Model file for the job. Use its own axes, mm. Face numbers are marked on the shaded views. A direction names the side the tool comes from. Round coordinates to 2 decimals unless told otherwise and drop trailing zeros. Order: outer loops, then holes, each group sorted by start corner. A loop starts at its lowest first (then second) coordinate and runs counter-clockwise, first axis right, second up. Notation, with made-up numbers: M 21,24 L 27,24 A9 cw 27,37 Z; hole C 60.5,3 d7. An arc over 180 degrees is marked long. Return JSON: item names as keys, results as strings. Group by question number.
Item 1: Probe line 1 along Y through (x, z) = (-6, 0); line 2 along X through (y, z) = (44, 25.5); line 3 along Y through (x, z) = (-37, -0.5). List the from-to ranges inside material, lowest first.
Item 2: Slice it at D-D on z = 40. Write the cut outline in (x, y), then the cut area to 3 significant figures.
Item 3: Slice it at C-C on y = 37.5. Write the cut outline in (x, z).
Item 4: Slice it at B-B on x = 0. Write the cut outline in (y, z), then the cut area to 3 significant figures.
Item 5: Slice it at A-A on z = 0. Write the cut outline in (x, y).
Item 6: Pin check, flat tips, straight feed: pin 1 Ø3 at (y, z) = (77.5, -16.5) entering from -X; pin 2 Ø1.5 at (x, z) = (39.5, -0.5) entering from -Y; pin 3 Ø2 at (y, z) = (43, 40) entering from -X; pin 4 Ø12 at (x, y) = (-25, 19.5) entering from +Z. Stop position of each tip, or through.
Item 7: Which spindle directions (+Z, -Z, +X, -X, +Y, -Y) get a long thin tool onto all of the face, cutting with end or side? Do the marked faces 1, 2, 3, 4 and 5. Say none if no direction does.
from build123d import *

# Parameters (mm, degrees)
SKETCH1_R           = 50
BOSS_EXTRUDE1_DEPTH = 10
SKETCH2_W           = 50
SKETCH2_H           = 75
BOSS_EXTRUDE2_DEPTH = 80
SKETCH3_R           = 25
CUT_EXTRUDE4_DEPTH  = 76
CUT_EXTRUDE5_DEPTH  = 76
CHAMFER1_SIZE       = 5


with BuildPart() as part:
    # Sketch1 → Boss-Extrude1 (new body)
    with BuildSketch(Plane(origin=(0, 0, 0), x_dir=(1, 0, 0), z_dir=(0, 1, 0))):
        Circle(SKETCH1_R)
    extrude(amount=BOSS_EXTRUDE1_DEPTH)

    # Sketch2 → Boss-Extrude2 (add)
    with BuildSketch(Plane(origin=(0, 10, 0), x_dir=(1, 0, 0), z_dir=(0, 1, 0))):
        Rectangle(SKETCH2_W, SKETCH2_H)
    extrude(amount=BOSS_EXTRUDE2_DEPTH)

    # Sketch3 → Cut-Extrude4 (cut, through all)
    with BuildSketch(Plane(origin=(25, 0, 0), x_dir=(0, 0, -1), z_dir=(1, 0, 0))):
        with Locations((0, 50)):
            Circle(SKETCH3_R)
    extrude(amount=-CUT_EXTRUDE4_DEPTH, mode=Mode.SUBTRACT)

    # Sketch4 → Cut-Extrude5 (cut, through all)
    with BuildSketch(Plane(origin=(25, 0, 0), x_dir=(0, 0, -1), z_dir=(1, 0, 0))):
        with BuildLine():
            Line((-37.5, 50), (-37.5, 90))
            Line((-37.5, 90), (37.5, 90))
            Line((37.5, 90), (37.5, 50))
            ThreePointArc((37.5, 50), (0, 87.5), (-37.5, 50))
        make_face()
    extrude(amount=-CUT_EXTRUDE5_DEPTH, mode=Mode.SUBTRACT)

    # Chamfer1
    chamfer1_edges = [part.edges().sort_by_distance(p)[0] for p in [
        (25, 30, 37.5),
        (-25, 30, 37.5),
        (-25, 30, -37.5),
        (25, 30, -37.5),
        (-25, 87.5, 0),
        (25, 87.5, 0),
    ]]
    chamfer(chamfer1_edges, length=CHAMFER1_SIZE)


solid = part.part
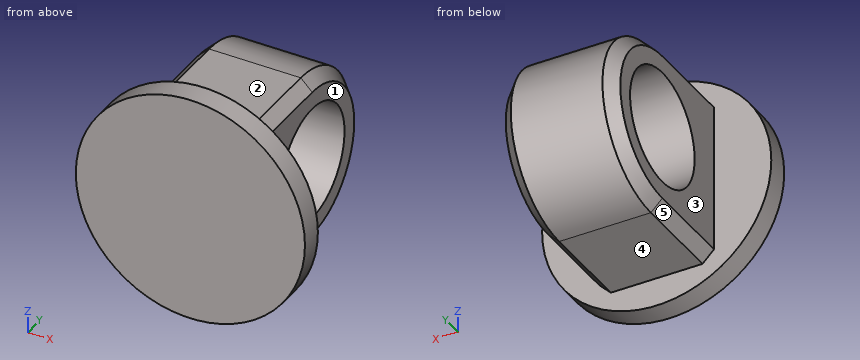
Output values:
{
 "1": {"line 1": "0 to 25, 75 to 87.5", "line 2": "-25 to 25", "line 3": "0 to 10"},
 "2": {"outline": "M -30,0 L 30,0 L 30,10 L -30,10 Z", "area": "600 mm²"},
 "3": {"outline": "M -25,-32.5 L -20,-37.5 L 20,-37.5 L 25,-32.5 L 25,-21.65 L -25,-21.65 Z; M -25,21.65 L 25,21.65 L 25,32.5 L 20,37.5 L -20,37.5 L -25,32.5 Z"},
 "4": {"outline": "M 0,-50 L 10,-50 L 10,-37.5 L 50,-37.5 A37.5 ccw 50,37.5 L 10,37.5 L 10,50 L 0,50 Z; hole C 50,0 d50", "area": "4,250 mm²"},
 "5": {"outline": "M -50,0 L 50,0 L 50,10 L 25,10 L 25,25 L -25,25 L -25,10 L -50,10 Z; M -25,75 L 25,75 L 25,82.5 L 20,87.5 L -20,87.5 L -25,82.5 Z"},
 "6": {"pin 1": "x = -25", "pin 2": "y = 0", "pin 3": "through", "pin 4": "z = 37.5"},
 "7": {"face 1": "+Z, -Z, +X, +Y", "face 2": "+Z, +X, -X, +Y", "face 3": "+Z, -Z, -X, +Y", "face 4": "-Z, +X, -X, +Y", "face 5": "-Z, -X, +Y"}
}
